The figure shows three views and two pictorial views of one solid part (mm, origin at its lowest corner). Answer the questions. A direction names the side the tool comes from. Coordinates: 2 decimals unless noted, no trailing zeros. Write each loop counter-clockwise with the first axis right and the second up, starting at its lowest first coordinate (ties: lowest second). Pieces come first, ordered by that corner, then holes.
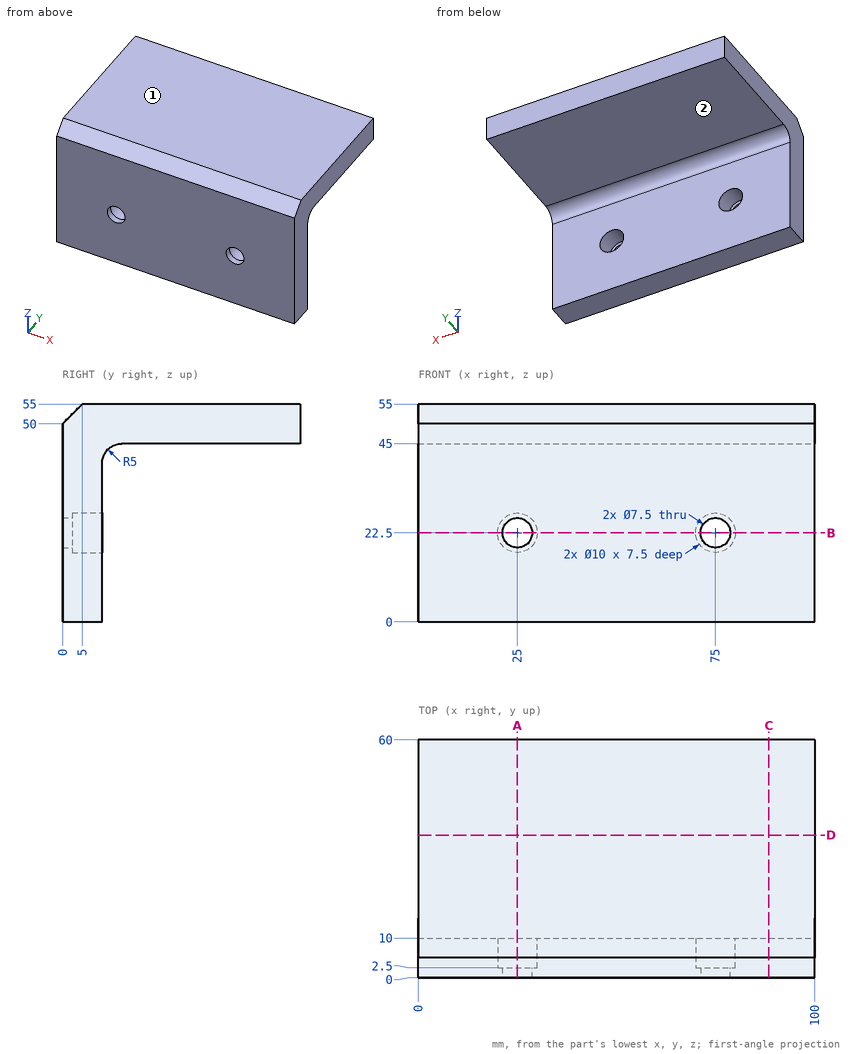
Q1. The part is cut by section B-B, the plane z = 22.5. Write down the section's boundary in (x, y).
Answers below:
outline: (0, 0) - (21.25, 0) - (21.25, 2.5) - (20, 2.5) - (20, 10) - (0, 10) - close; (28.75, 0) - (71.25, 0) - (71.25, 2.5) - (70, 2.5) - (70, 10) - (30, 10) - (30, 2.5) - (28.75, 2.5) - close; (78.75, 0) - (100, 0) - (100, 10) - (80, 10) - (80, 2.5) - (78.75, 2.5) - close
Q2. Which of the six approach directions +Z, -Z, +X, -X, +Y, -Y give full straight-line access (tool end or side, diameter ignored) to the marked faces 1 and 2?
Answers below:
face 1: +Z, +X, -X, +Y, -Y
face 2: -Z, +X, -X, +Y
Q3. Find the intervals of material crossed by probe 1 along X at (y, z) = (8, 22); probe 2 along Z at (x, y) = (75, 6.5); probe 3 along Z at (x, y) = (38, 18.5), in increasing order.
Answers below:
probe 1: x = 0 to 20.03, 29.97 to 70.03, 79.97 to 100
probe 2: z = 0 to 17.5, 27.5 to 55
probe 3: z = 45 to 55
Q4. The part is cut by section A-A, the plane x = 25. Write down the section's boundary in (y, z).
Answers below:
outline: (0, 0) - (10, 0) - (10, 17.5) - (2.5, 17.5) - (2.5, 18.75) - (0, 18.75) - close; (0, 26.25) - (2.5, 26.25) - (2.5, 27.5) - (10, 27.5) - (10, 40) arc R5 cw to (15, 45) - (60, 45) - (60, 55) - (5, 55) - (0, 50) - close
Q5. The part is cut by section C-C, the plane x = 88.5. Write down the section's boundary in (y, z), then the cut area to 3 significant figures.
Answers below:
outline: (0, 0) - (10, 0) - (10, 40) arc R5 cw to (15, 45) - (60, 45) - (60, 55) - (5, 55) - (0, 50) - close
area: 1,040 mm2
Q6. Given pin 1 (8.5 mm diameter, centred on x = 25, z = 22.5, fed in from +Y); pin 2 (22.5 mm diameter, centred on x = 41.5, y = 40, fed in from -Z); pin 3 (10 mm diameter, centred on x = 24.5, z = 25.5, fed in from +Y), each flat-ended and moving along its own axis, determine where each tip first touches the part or whether it passes through.
Answers below:
pin 1: stops at y = 2.5
pin 2: stops at z = 45
pin 3: stops at y = 10
Q7. The part is cut by section D-D, the plane y = 36. Write down the section's boundary in (x, z).
Answers below:
outline: (0, 45) - (100, 45) - (100, 55) - (0, 55) - close
